Work out the finished part from the listing and answer in its coordinate system (mm). Face numbers are marked on the shaded views. Coordinates: 2 decimals unless noted, no trailing zeros. Loops run counter-clockwise (first coordinate to the right, second up) from the corner with the lowest first, then second, coordinate; pieces in that order, holes last. Notation, with made-up numbers: (60, 83) - (71, 83) arc R23 ccw to (71, 105) - close; hole circle Ø3 at (43.25, 55.25). An arc over 180 degrees is marked (long way). Write each question's results on one line, items separated by ' | '. Start each with the question number.
1. A cutting plane is placed at A-A on x = 12.8. Determine the outline of the cut face in (y, z), then the cut area to 3 significant figures.
2. Find the intervals of material crossed by line 1 along Y through (x, z) = (32.8, 4.15); line 2 along X through (y, z) = (15, 5.65); line 3 along X through (y, z) = (-2, 5), in increasing order. Write a range as [from, to].
3. This flat-tipped pin is pushed along its axis until it touches: P1, Ø4, axis at x = 12.8, y = 10, coming from the +Z side. Where does it stop, or does it pass through?
4. Determine the mould class of the marked faces 1, 2, 3 and 4 for opening direction X: released by +X, released by -X, zero draft, split by the parting line, or undercut.
5. A cutting plane is placed at B-B on y = 1. Determine the outline of the cut face in (x, z), then the cut area to 3 significant figures.
6. A cutting plane is placed at D-D on x = -14. Determine the outline of the cut face in (y, z).
7. A cutting plane is placed at C-C on z = 4.6. State how many separate pieces and enclosed holes the cut face has, then the cut area to 3 significant figures.
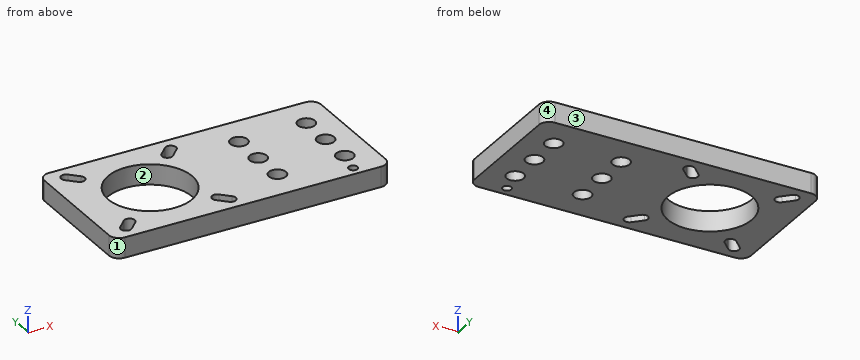
from build123d import *

# Parameters (mm, degrees)
F0_R     = 12.5
F0_R_2   = 2.55
F0_R_3   = 1.3
F1_DEPTH = 6


# Not quite as in the source:
# - ends of sketch curves that miss each other by under 0.0002 mm in the source are joined


with BuildPart() as f1:
    # F0 (on Top) → F1 (new body)
    with BuildSketch(Plane.XY):
        with BuildLine():
            Line((38, 19.75), (-38, 19.75))
            ThreePointArc((-38, 19.75), (-40.1213203436, 18.8713203436), (-41, 16.75))
            Line((-41, 16.75), (-41, -16.75))
            ThreePointArc((-41, -16.75), (-40.1213203436, -18.8713203436), (-38, -19.75))
            Line((-38, -19.75), (38, -19.75))
            ThreePointArc((38, -19.75), (40.1213203436, -18.8713203436), (41, -16.75))
            Line((41, -16.75), (41, 16.75))
            ThreePointArc((41, 16.75), (40.1213203436, 18.8713203436), (38, 19.75))
        make_face()
        with BuildLine():
            ThreePointArc((-34.1539839892, -16.5960150108), (-36.3460155108, -16.5960155108), (-36.3460150108, -14.4039839892))
            Line((-36.346015, -14.403984), (-33.846015, -11.903984))
            ThreePointArc((-33.8460150108, -11.9039839892), (-31.6539844892, -11.9039844892), (-31.6539839892, -14.0960150108))
            Line((-31.653984, -14.096015), (-34.153984, -16.596015))
        make_face(mode=Mode.SUBTRACT)
        with BuildLine():
            ThreePointArc((-3.1539844892, -14.4039844892), (-3.1539844892, -16.5960155108), (-5.3460155108, -16.5960155108))
            Line((-5.3460155108, -16.5960155108), (-7.846015, -14.096015))
            ThreePointArc((-7.846015, -14.096015), (-7.8460155108, -11.9039844892), (-5.6539844892, -11.9039844892))
            Line((-5.6539844892, -11.9039844892), (-3.1539844892, -14.4039844892))
        make_face(mode=Mode.SUBTRACT)
        with Locations((-19.25, 0)):
            Circle(F0_R, mode=Mode.SUBTRACT)
        with Locations((12.8, -10)):
            Circle(F0_R_2, mode=Mode.SUBTRACT)
        with Locations((31.4, -16.75)):
            Circle(F0_R_3, mode=Mode.SUBTRACT)
        with Locations((32.8, -10)):
            Circle(F0_R_2, mode=Mode.SUBTRACT)
        with Locations((12.8, 0)):
            Circle(F0_R_2, mode=Mode.SUBTRACT)
        with Locations((32.8, 0)):
            Circle(F0_R_2, mode=Mode.SUBTRACT)
        with BuildLine():
            ThreePointArc((-31.6539844892, 14.0960155108), (-31.6539844892, 11.9039844892), (-33.8460155108, 11.9039844892))
            Line((-33.8460155108, 11.9039844892), (-36.346015, 14.403985))
            ThreePointArc((-36.346015, 14.403985), (-36.3460155108, 16.5960155108), (-34.1539844892, 16.5960155108))
            Line((-34.1539844892, 16.5960155108), (-31.6539844892, 14.0960155108))
        make_face(mode=Mode.SUBTRACT)
        with BuildLine():
            ThreePointArc((-5.3460150108, 16.5960160108), (-3.1539844892, 16.5960155108), (-3.1539839892, 14.4039849892))
            Line((-3.153984, 14.403985), (-5.653984, 11.903985))
            ThreePointArc((-5.6539839892, 11.9039849892), (-7.8460155108, 11.9039844892), (-7.8460150108, 14.0960160108))
            Line((-7.846015, 14.096016), (-5.346015, 16.596016))
        make_face(mode=Mode.SUBTRACT)
        with Locations((12.8, 10)):
            Circle(F0_R_2, mode=Mode.SUBTRACT)
        with Locations((32.8, 10)):
            Circle(F0_R_2, mode=Mode.SUBTRACT)
    extrude(amount=F1_DEPTH)


solid = f1.part
Values:
1) outline: (-19.75, 0) - (-12.55, 0) - (-12.55, 6) - (-19.75, 6) - close; (-7.45, 0) - (-2.55, 0) - (-2.55, 6) - (-7.45, 6) - close; (2.55, 0) - (7.45, 0) - (7.45, 6) - (2.55, 6) - close; (12.55, 0) - (19.75, 0) - (19.75, 6) - (12.55, 6) - close | area: 145 mm^2
2) line 1: [-19.75, -12.55], [-7.45, -2.55], [2.55, 7.45], [12.55, 19.75] | line 2: [-41, -36.72], [-32.56, -6.94], [-2.78, 41] | line 3: [-41, -31.59], [-6.91, 11.22], [14.38, 31.22], [34.38, 41]
3) P1: through
4) face 1: released by -X | face 2: undercut | face 3: zero draft | face 4: released by +X
5) outline: (-41, 0) - (-31.71, 0) - (-31.71, 6) - (-41, 6) - close; (-6.79, 0) - (10.45, 0) - (10.45, 6) - (-6.79, 6) - close; (15.15, 0) - (30.45, 0) - (30.45, 6) - (15.15, 6) - close; (35.15, 0) - (41, 0) - (41, 6) - (35.15, 6) - close | area: 286 mm^2
6) outline: (-19.75, 0) - (-11.34, 0) - (-11.34, 6) - (-19.75, 6) - close; (11.34, 0) - (19.75, 0) - (19.75, 6) - (11.34, 6) - close
7) separate pieces: 1 | enclosed holes: 12 | area: 2,540 mm^2
